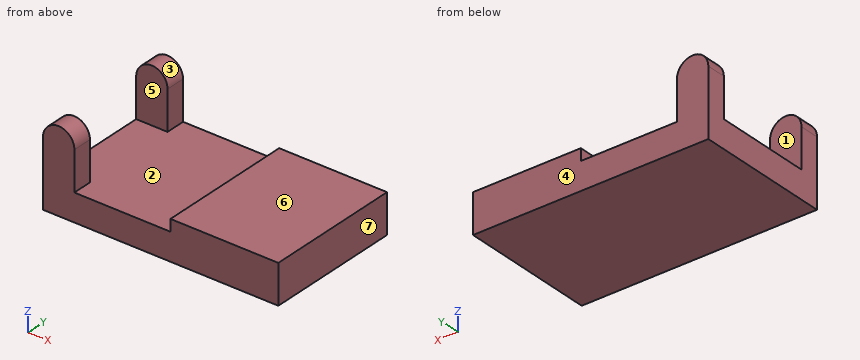
from build123d import *

# Parameters (mm, degrees)
F0_W     = 120
F0_H     = 70
F1_DEPTH = 20
F2_W     = 65
F2_H     = 6
F3_DEPTH = 100
F5_DEPTH = 10
F7_DEPTH = 10


with BuildPart() as f1:
    # F0 (on Top) → F1 (new body)
    with BuildSketch(Plane.XY):
        Rectangle(F0_W, F0_H)
    extrude(amount=F1_DEPTH)

    # F2 (on face) → F3 (cut)
    with BuildSketch(Plane.XZ.offset(35)):
        with Locations((-27.5, 17)):
            Rectangle(F2_W, F2_H)
    extrude(amount=-F3_DEPTH, mode=Mode.SUBTRACT)

    # F4 (on face) → F5 (join)
    with BuildSketch(Plane.XZ.offset(35)):
        with BuildLine():
            ThreePointArc((-44, 34), (-52, 42), (-60, 34))
            Line((-60, 34), (-44, 34))
        make_face()
        with BuildLine():
            Line((-44, 34), (-60, 34))
            ThreePointArc((-60, 34), (-52, 26), (-44, 34))
        make_face()
        with BuildLine():
            Line((-60, 34), (-60, 14))
            Line((-60, 14), (-44, 14))
            Line((-44, 14), (-44, 34))
            ThreePointArc((-44, 34), (-52, 26), (-60, 34))
        make_face()
    extrude(amount=-F5_DEPTH)

    # F6 (on face) → F7 (join)
    with BuildSketch(Plane(origin=(0, 35, 0), x_dir=(-1, 0, 0), z_dir=(0, 1, 0))):
        with BuildLine():
            Line((44, 14), (60, 14))
            Line((60, 14), (60, 34))
            ThreePointArc((60, 34), (52, 26), (44, 34))
            Line((44, 34), (44, 14))
        make_face()
        with BuildLine():
            ThreePointArc((44, 34), (52, 26), (60, 34))
            Line((60, 34), (44, 34))
        make_face()
        with BuildLine():
            Line((44, 34), (60, 34))
            ThreePointArc((60, 34), (52, 42), (44, 34))
        make_face()
    extrude(amount=-F7_DEPTH)


solid = f1.part
Source: CAD feature listing. Evaluate the final solid. Frame: model axes, mm. Face numbers are marked on the shaded views. A direction names the side the tool comes from. Coordinates: 2 decimals unless noted, no trailing zeros. Order: outer loops, then holes, each group sorted by start corner. A loop starts at its lowest first (then second) coordinate and runs counter-clockwise, first axis right, second up. Notation, with made-up numbers: M 83.5,23.25 L 91.5,23.25 A33 cw 91.5,52.25 Z; hole C 43,48 d8. An arc over 180 degrees is marked long. Write each question's results on one line, items separated by ' | '. Start each with the question number.
Item 1: Draft query along Y for the marked faces 1, 2, 3 and 4. Return one class per face: pulls with the +Y half, pulls with the -Y half, needs draft (parallel to the pull), parting line crosses it, or undercut.
Item 2: Cut plane D-D (y = -18.5). Return loops of the section in (x, z), and give its area (3 significant figures).
Item 3: Cut plane B-B (z = 27.5). Return loops of the section in (x, y).
Item 4: Set-up query: the marked faces 5, 6 and 7. Return all of +Z, -Z, +X, -X, +Y, -Y with unobstructed straight access to the full face (end or side cutting, diameter ignored); none if empty.
Item 5: Cut plane C-C (x = -52). Return loops of the section in (y, z), and give its area (3 significant figures).
Item 6: First-contact query: pin 1 Ø12 at (x, y) = (-30, -1.5) entering from +Z; pin 2 Ø3 at (y, z) = (-22, 17.5) entering from -X; pin 3 Ø3 at (y, z) = (-32, 28) entering from +X. Flat tips, straight axial feed; report the tip coordinate or a pass-through.
Item 7: Cut plane A-A (z = 18.5). Return loops of the section in (x, y).
Item 8: Line query: probe 1 along Z at (x, y) = (9, -6.5); probe 2 along Z at (x, y) = (-19, 30.5); probe 3 along X at (y, z) = (14.5, 19.5). Output: solid intervals per line, ascending.
Checked values:
1) face 1: undercut | face 2: undercut | face 3: needs draft | face 4: pulls with the +Y half
2) outline: M -60,0 L 60,0 L 60,20 L 5,20 L 5,14 L -60,14 Z | area: 2,010 mm2
3) outline: M -60,-35 L -44,-35 L -44,-25 L -60,-25 Z; M -60,25 L -44,25 L -44,35 L -60,35 Z
4) face 5: +Z, -X | face 6: +Z, +X, +Y, -Y | face 7: +Z, -Z, +X, +Y, -Y
5) outline: M -35,0 L 35,0 L 35,42 L 25,42 L 25,14 L -25,14 L -25,42 L -35,42 Z | area: 1,540 mm2
6) pin 1: stops at z = 14 | pin 2: stops at x = 5 | pin 3: stops at x = -44
7) outline: M -60,-35 L -44,-35 L -44,-25 L -60,-25 Z; M -60,25 L -44,25 L -44,35 L -60,35 Z; M 5,-35 L 60,-35 L 60,35 L 5,35 Z
8) probe 1: z = 0 to 20 | probe 2: z = 0 to 14 | probe 3: x = 5 to 60
